Geometry: see drawing. Coordinates: mm, zero at the bounding-box minimum. A direction names the side the tool comes from. Round coordinates to 2 decimals unless told otherwise and drop trailing zeros. Loops run counter-clockwise (first coordinate to the right, second up) from the corner with the lowest first, then second, coordinate; pieces in that order, holes last. Notation, with made-up numbers: (41, -26.5) - (100, -26.5) arc R20 ccw to (100, -8.5) - close; hole circle Ø3 at (-14.75, -29.5). An arc over 180 degrees is marked (long way). Use CSV: the item, a comma, the result in double quotes.
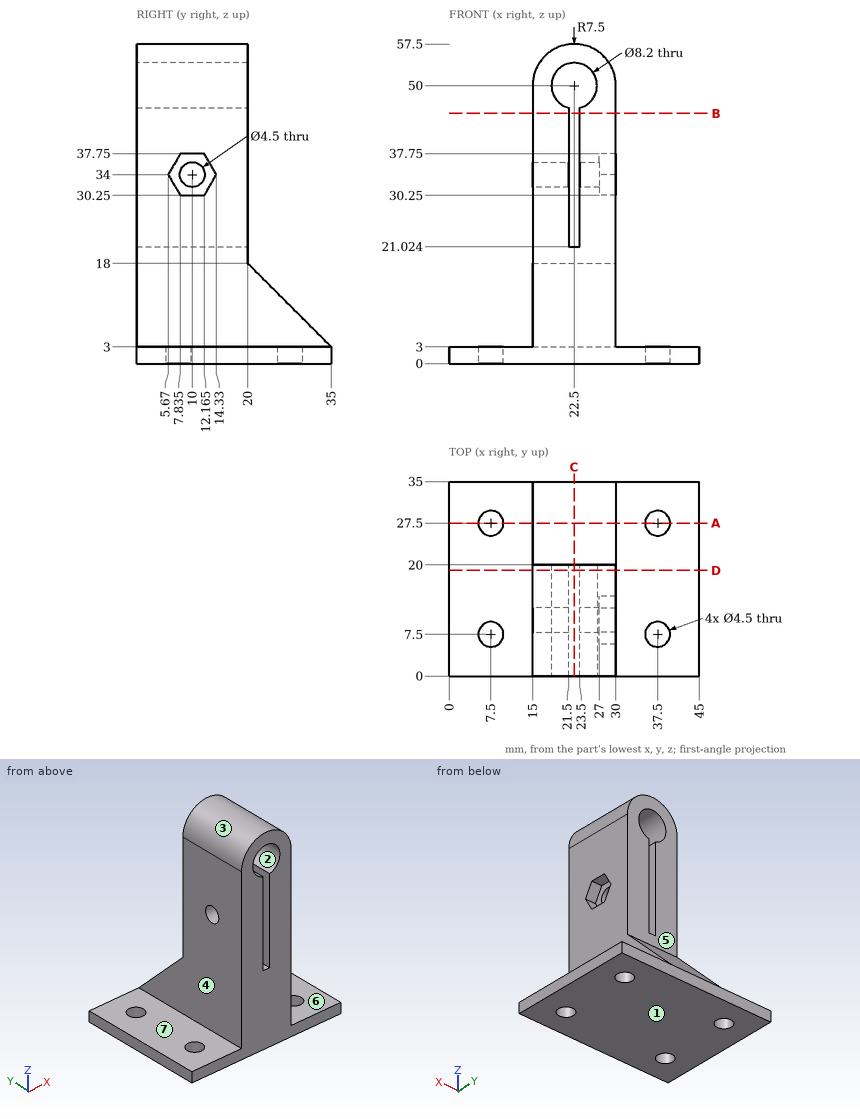
Item 1: Mould query, pull axis X, two halves, no side actions, for the marked faces 1, 2, 3 and 4. Classes: released by +X, released by -X, zero draft, split by the parting line, or undercut.
Final values:
face 1,"zero draft"
face 2,"undercut"
face 3,"split by the parting line"
face 4,"released by -X"
Item 2: Reachability of the marked faces 5, 6 and 7 from +Z, -Z, +X, -X, +Y, -Y: full face, straight path, thin tool, end or side. Return the list, or none.
Final values:
face 5,"+Z, +X, -X, +Y"
face 6,"+Z, +X, +Y, -Y"
face 7,"+Z, -X, +Y, -Y"
Item 3: Section C-C on x = 22.5. Return the cut outline in (y, z), plus the area to 3 significant figures.
Final values:
outline,"(0, 0) - (35, 0) - (35, 3) - (20, 18) - (20, 21.02) - (0, 21.02) - close; (0, 54.1) - (20, 54.1) - (20, 57.5) - (0, 57.5) - close"
area,"646 mm²"
Item 4: Section A-A on y = 27.5. Return the cut outline in (x, z), plus the area to 4 significant figures.
Final values:
outline,"(0, 0) - (5.25, 0) - (5.25, 3) - (0, 3) - close; (9.75, 0) - (35.25, 0) - (35.25, 3) - (30, 3) - (30, 10.5) - (15, 10.5) - (15, 3) - (9.75, 3) - close; (39.75, 0) - (45, 0) - (45, 3) - (39.75, 3) - close"
area,"220.5 mm²"
Item 5: Section B-B on z = 45. Return the cut outline in (x, y), plus the area to 3 significant figures.
Final values:
outline,"(15, 0) - (21.5, 0) - (21.5, 20) - (15, 20) - close; (23.5, 0) - (30, 0) - (30, 20) - (23.5, 20) - close"
area,"260 mm²"
Item 6: Pin query (flat end, axial travel): P1, Ø10, axis at y = 14.5, z = 28, coming from the -X side; P2, Ø3.5, axis at x = 37.5, y = 7.5, coming from the -Z side; P3, Ø12, axis at y = 24.5, z = 24, coming from the +X side; P4, Ø16.5, axis at x = 25.5, z = 40, coming from the +Y side. Return the tip coordinate at first contact, or that it passes through.
Final values:
P1,"stops at x = 15"
P2,"passes through"
P3,"stops at x = 30"
P4,"stops at y = 20"
Item 7: Material intervals for line 1 (Y direction, x = 7.5, z = 1.7); line 2 (X direction, y = 7, z = 2); line 3 (X direction, y = 14, z = 36), sorted ascending.
Final values:
line 1,"y = 0 to 5.25, 9.75 to 25.25, 29.75 to 35"
line 2,"x = 0 to 5.31, 9.69 to 35.31, 39.69 to 45"
line 3,"x = 15 to 21.5, 23.5 to 30"
Item 8: Section D-D on y = 19. Return the cut outline in (x, z).
Final values:
outline,"(0, 0) - (45, 0) - (45, 3) - (30, 3) - (30, 50) arc R7.5 ccw to (15, 50) - (15, 3) - (0, 3) - close; hole (21.5, 21.02) - (23.5, 21.02) - (23.5, 46.02) arc R4.1 ccw (long way) to (21.5, 46.02) - close"
